Check sheet for the modelled part. Datum: model origin and axes. Units: mm. A direction names the side the tool comes from. Coordinates: 2 decimals unless noted, no trailing zeros. Order: outer loops, then holes, each group sorted by start corner. A loop starts at its lowest first (then second) coordinate and runs counter-clockwise, first axis right, second up. Notation, with made-up numbers: (16.25, 27.25) -> (60.25, 27.25) arc R20 cw to (60.25, 49.25) -> close; hole circle Ø3 at (49, 24). An arc over 180 degrees is marked (long way). Put each result on its own line as item: value. Start each with the question number.
```python
from build123d import *

# Parameters (mm, degrees)
SKETCH1_R           = 1.55
SKETCH1_W           = 61.4
SKETCH1_H           = 66.34
BOSS_EXTRUDE1_DEPTH = 2
BOSS_EXTRUDE2_DEPTH = 16.5
FILLET1_R           = 7.5
SKETCH3_R           = 1.55
CUT_EXTRUDE1_DEPTH  = 10


with BuildPart() as part:
    # Sketch1 → Boss-Extrude1 (new body)
    # profile 1 of 2: a face of its own
    with BuildSketch(Plane(origin=(0, 0, 0), x_dir=(1, 0, 0), z_dir=(0, 1, 0))):
        Polygon((42.27964617, -55.129137945), (42.27964617, -47.129137945), (64.04371989, -47.129137945), (64.04371989, -55.129137945), (110.09964617, -55.129137945), (110.09964617, -91.329137945), (-3.55035383, -91.329137945), (-3.55035383, -55.129137945), align=None)
        with Locations(Location((46.27964617, -51.129137945, 0), (0, 0, 270))):
            Circle(SKETCH1_R, mode=Mode.SUBTRACT)
        with Locations(Location((60.04371989, -51.129137945, 0), (0, 0, 270))):
            Circle(SKETCH1_R, mode=Mode.SUBTRACT)
    # profile 2 of 2: a face of its own
    with BuildSketch(Plane(origin=(0, 0, 0), x_dir=(1, 0, 0), z_dir=(0, 1, 0))):
        with Locations((53.27464617, -88.299137945)):
            Rectangle(SKETCH1_W, SKETCH1_H)
    extrude(amount=BOSS_EXTRUDE1_DEPTH)

    # Sketch2 → Boss-Extrude2 (add)
    with BuildSketch(Plane(origin=(0, 2, 0), x_dir=(1, 0, 0), z_dir=(0, 1, 0))):
        Polygon((22.57464617, -91.329137945), (22.57464617, -121.469137945), (52.02464617, -121.469137945), (52.02464617, -119.469137945), (24.57464617, -119.469137945), (24.57464617, -57.129137945), (81.97464617, -57.129137945), (81.97464617, -119.469137945), (54.52464617, -119.469137945), (54.52464617, -121.469137945), (83.97464617, -121.469137945), (83.97464617, -91.329137945), (83.97464617, -55.129137945), (64.04371989, -55.129137945), (42.27964617, -55.129137945), (22.57464617, -55.129137945), align=None)
    extrude(amount=BOSS_EXTRUDE2_DEPTH)

    # Fillet1
    fillet1_edges = [part.edges().sort_by_distance(p)[0] for p in [
        (81.97464617, 10.25, 119.469137945),
        (24.57464617, 10.25, 119.469137945),
        (24.57464617, 10.25, 57.129137945),
        (81.97464617, 10.25, 57.129137945),
    ]]
    fillet(fillet1_edges, radius=FILLET1_R)

    # Sketch3 → Cut-Extrude1 (cut)
    with BuildSketch(Plane(origin=(0, 18.5, 0), x_dir=(1, 0, 0), z_dir=(0, 1, 0))):
        with Locations(Location((24.82464617, -57.379137945, 0), (0, 0, 270))):
            Circle(SKETCH3_R)
        with Locations(Location((81.72464617, -57.379137945, 0), (0, 0, 90))):
            Circle(SKETCH3_R)
        with Locations(Location((81.72464617, -119.219137945, 0), (0, 0, 270))):
            Circle(SKETCH3_R)
        with Locations(Location((24.82464617, -119.219137945, 0), (0, 0, 90))):
            Circle(SKETCH3_R)
    extrude(amount=-CUT_EXTRUDE1_DEPTH, mode=Mode.SUBTRACT)


solid = part.part
```
1) Access from +Z, -Z, +X, -X, +Y, -Y to the whole of each face (thin tool, end or side, straight path). Record for faces 3 (the cylindrical face through (60.509, 0.986, 52.608)), 4 (the cylindrical face through (26.8, 10.4, 59.3)), 5 (the flat face through (9, 2, 73)), 6 (the flat face through (53, 2, 51)).
2) Scan lines: line 1 along X through (y, z) = (12, 109.5); line 2 along Z through (x, y) = (65.5, 13); line 3 along X through (y, z) = (16.25, 118.5). Record each from-to range of solid material in increasing order. Write a range as [from, to].
3) Mould release check, pull along X, two halves, no side actions. Record for faces 1 (the flat face through (81.975, 10, 88)), 2 (the flat face through (97, 2, 73)): +X half, -X half, draft (parallel to the pull), parting line (faces both ways), or undercut.
4) Sectioned sample at C-C (y = 4). Record the boundary of the cut face in (x, z).
5) Gauge pin test, flat ends, axial feed: pin 1 (0.6 mm diameter, centred on x = 101, y = 0.5, fed in from +Z); pin 2 (3 mm diameter, centred on y = 13, z = 111.5, fed in from -X); pin 3 (2 mm diameter, centred on x = 48.5, y = 12, fed in from -Z); pin 4 (1.9 mm diameter, centred on x = 46.28, z = 51.13, fed in from -Y). Record the tip position at first contact, or that the pin passes through.
6) Sectioned sample at D-D (x = 15.5). Record the boundary of the cut face in (y, z).
7) Sectioned sample at B-B (y = 17.25). Record the boundary of the cut face in (x, z).
8) Sectioned sample at A-A (z = 72). Record the boundary of the cut face in (x, y), plus the area to 3 significant figures.
Entries:
1. face 3: +Y, -Y
1. face 4: +Y
1. face 5: +Z, -Z, -X, +Y
1. face 6: -Z, +X, -X, +Y
2. line 1: x = [22.57, 24.57], [81.97, 83.97]
2. line 2: z = [55.13, 57.13], [119.47, 121.47]
2. line 3: x = [22.57, 23.45], [26.2, 28.39], [78.16, 80.35], [83.1, 83.97]
3. face 1: undercut
3. face 2: draft
4. outline: (22.57, 55.13) -> (83.97, 55.13) -> (83.97, 121.47) -> (54.52, 121.47) -> (54.52, 119.47) -> (74.47, 119.47) arc R7.5 cw to (81.97, 111.97) -> (81.97, 64.63) arc R7.5 cw to (74.47, 57.13) -> (32.07, 57.13) arc R7.5 cw to (24.57, 64.63) -> (24.57, 111.97) arc R7.5 cw to (32.07, 119.47) -> (52.02, 119.47) -> (52.02, 121.47) -> (22.57, 121.47) -> close
5. pin 1: stops at z = 91.33
5. pin 2: stops at x = 22.57
5. pin 3: stops at z = 55.13
5. pin 4: passes through
6. outline: (0, 55.13) -> (2, 55.13) -> (2, 91.33) -> (0, 91.33) -> close
7. outline: (22.57, 55.13) -> (83.97, 55.13) -> (83.97, 121.47) -> (54.52, 121.47) -> (54.52, 119.47) -> (74.47, 119.47) arc R7.5 cw to (81.97, 111.97) -> (81.97, 64.63) arc R7.5 cw to (74.47, 57.13) -> (32.07, 57.13) arc R7.5 cw to (24.57, 64.63) -> (24.57, 111.97) arc R7.5 cw to (32.07, 119.47) -> (52.02, 119.47) -> (52.02, 121.47) -> (22.57, 121.47) -> close; hole circle Ø3.1 at (24.82, 57.38); hole circle Ø3.1 at (24.82, 119.22); hole circle Ø3.1 at (81.72, 57.38); hole circle Ø3.1 at (81.72, 119.22)
8. outline: (-3.55, 0) -> (110.1, 0) -> (110.1, 2) -> (83.97, 2) -> (83.97, 18.5) -> (81.97, 18.5) -> (81.97, 2) -> (24.57, 2) -> (24.57, 18.5) -> (22.57, 18.5) -> (22.57, 2) -> (-3.55, 2) -> close
8. area: 293 mm2
